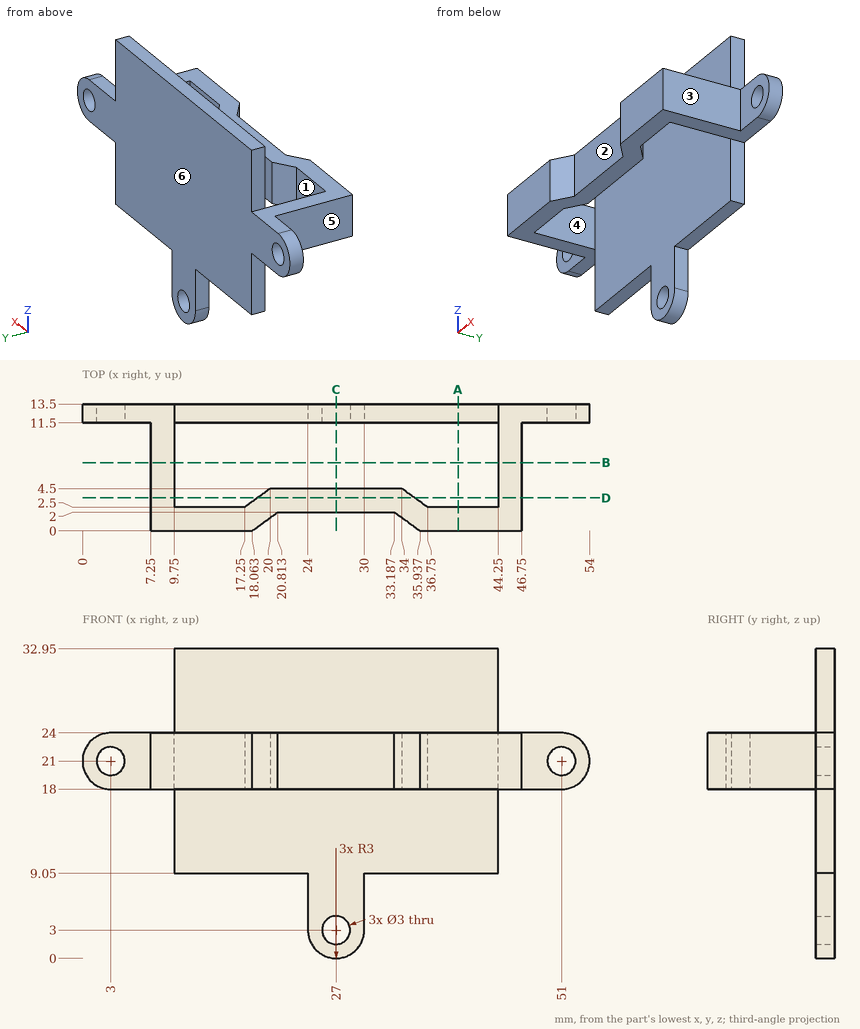
Verification items for this drawing (mm, ordinates from the low corner). A direction names the side the tool comes from. Coordinates: 2 decimals unless noted, no trailing zeros. Loops run counter-clockwise (first coordinate to the right, second up) from the corner with the lowest first, then second, coordinate; pieces in that order, holes last. Notation, with made-up numbers: (54, -27.5) - (79, -27.5) arc R19 ccw to (79, -5.5) - close; hole circle Ø10 at (71.5, 39.5). An arc over 180 degrees is marked (long way). Use one line per item in the form item = value. Start each with the question number.
Item 1: Section check B-B, the plane y = 7.25. Enter the section's corners in (x, z), and give its area (3 significant figures).
Item 2: Tool access check on the marked faces 1, 2 and 3. Record the directions out of +Z, -Z, +X, -X, +Y, -Y that give a thin tool (end or side, any length) a straight path to the whole face; none if there is none.
Item 3: Gauge pin test, flat ends, axial feed: pin 1 (1.8 mm diameter, centred on x = 51, z = 21, fed in from -Y); pin 2 (7 mm diameter, centred on x = 27, y = 5, fed in from -Z); pin 3 (5 mm diameter, centred on x = 14, y = 3, fed in from +Z); pin 4 (2 mm diameter, centred on y = 12, z = 6.5, fed in from -X). Record the tip position at first contact, or that the pin passes through.
Item 4: Thickness scan on probe 1 along Z at (x, y) = (3, 12.05); probe 2 along X at (y, z) = (3.25, 19); probe 3 along X at (y, z) = (5.25, 21.5). Record the ranges inside material, lowest first.
Item 5: Mould release check, pull along Y, two halves, no side actions. Record for the marked faces 4, 5 and 6: +Y half, -Y half, draft (parallel to the pull), parting line (faces both ways), or undercut.
Item 6: Section check A-A, the plane x = 40. Enter the section's corners in (y, z), and give its area (3 significant figures).
Item 7: Section check C-C, the plane x = 27. Enter the section's corners in (y, z).
Item 8: Section check D-D, the plane y = 3.5. Enter the section's corners in (x, z) (3 decimals).
Computed:
q1.outline = (7.25, 18) - (9.75, 18) - (9.75, 24) - (7.25, 24) - close; (44.25, 18) - (46.75, 18) - (46.75, 24) - (44.25, 24) - close
q1.area = 30.0 mm2
q2.face_1 = +Z, -Z
q2.face_2 = +Z, -Z, -Y
q2.face_3 = +Z, -Z, +X, -Y
q3.pin_1 = through
q3.pin_2 = 18
q3.pin_3 = 24
q3.pin_4 = 24
q4.probe_1 = 18 to 19.5, 22.5 to 24
q4.probe_2 = 7.25 to 9.75, 18.28 to 35.72, 44.25 to 46.75
q4.probe_3 = 7.25 to 9.75, 44.25 to 46.75
q5.face_4 = undercut
q5.face_5 = draft
q5.face_6 = +Y half
q6.outline = (0, 18) - (2.5, 18) - (2.5, 24) - (0, 24) - close; (11.5, 9.05) - (13.5, 9.05) - (13.5, 32.95) - (11.5, 32.95) - close
q6.area = 62.8 mm2
q7.outline = (2, 18) - (4.5, 18) - (4.5, 24) - (2, 24) - close; (11.5, 0) - (13.5, 0) - (13.5, 1.5) - (11.5, 1.5) - close; (11.5, 4.5) - (13.5, 4.5) - (13.5, 32.95) - (11.5, 32.95) - close
q8.outline = (7.25, 18) - (9.75, 18) - (9.75, 24) - (7.25, 24) - close; (18.625, 18) - (35.375, 18) - (35.375, 24) - (18.625, 24) - close; (44.25, 18) - (46.75, 18) - (46.75, 24) - (44.25, 24) - close
